Autodesk Inventor part; units mm, degrees
ref_plane "YZ Plane" through (0, 0, 0) normal (1, 0, 0) x (0, 1, 0)
ref_plane "XZ Plane" through (0, 0, 0) normal (0, 1, 0) x (-1, 0, 0)
ref_plane "XY Plane" through (0, 0, 0) normal (0, 0, 1) x (1, 0, 0)
sketch "Sketch1" plane through (0, 0, 0) normal (0, 1, 0) x (-1, 0, 0)
  line L0 (110, -125) -> (-110, -125)
  line L1 (-110, -125) -> (-110, 125)
  line L2 (-110, 125) -> (110, 125)
  line L3 (110, 125) -> (110, -125)
  line L4 (110, -125) -> (-110, 125) construction
  line L5 (-110, -125) -> (110, 125) construction
  line L6 (-60, 75) -> (60, 75) construction
  line L7 (60, 75) -> (60, -75) construction
  line L8 (60, -75) -> (-60, -75) construction
  line L9 (-60, -75) -> (-60, 75) construction
  line L10 (-60, 75) -> (60, -75) construction
  line L11 (60, 75) -> (-60, -75) construction
  point P0 (0, 0)
  dimension "d0" = 220
  dimension "d1" = 250
  dimension "d2" = 120
  dimension "d3" = 150
extrude "Extrusion1" add sketch "Sketch1" along normal blind 40
hole "Hole1" at (-60, 0, -75) at (60, 0, -75) at (60, 0, 75) at (-60, 0, 75) direction (0, 1, 0) diameter 8 end through all
sketch "Sketch2" plane through (-110, 0, 125) normal (0, 0, 1) x (1, 0, 0)
  line L0 (0, 0) -> (220, 0) construction
  line L1 (0, 40) -> (220, 40) construction
  line L2 (220, 0) -> (0, 40) construction
  line L3 (0, 0) -> (220, 40) construction
  circle A0 centre (110, 20) radius 15
  point P0 (110, 0)
  dimension "d13" = 30
extrude "Extrusion2" cut sketch "Sketch2" against normal through all
properties part number "SACMI DPA TILES GRIP FIXED SUPPORT"
Geometry check sheet. Reference: the model listing, model coordinates, mm. Coordinates: 2 decimals unless noted, no trailing zeros. Order: outer loops, then holes, each group sorted by start corner. A loop starts at its lowest first (then second) coordinate and runs counter-clockwise, first axis right, second up. Notation, with made-up numbers: (-31.5, 32.25) -> (18.5, 32.25) arc R26 ccw to (18.5, 49.25) -> close; hole circle Ø2 at (30.25, 18.25). An arc over 180 degrees is marked (long way). Use a Markdown table: item, result. Add a question column.
1. Cross-section at A-A (y = 20). Enter the section's corners in (x, z).
2. Cross-section at B-B (z = 75). Enter the section's corners in (x, y), and give its area (3 significant figures).
3. Mould release check, pull along X, two halves, no side actions. Record for faces 1 (the face through (2, 40, 2)), 2 (the face through (63.905, 20.28, -74.133)), 3 (the face through (-110, 20, 2)): pulls with the +X half, pulls with the -X half, needs draft (parallel to the pull), parting line crosses it, or undercut.
4. Cross-section at C-C (x = -60). Enter the section's corners in (y, z).
5. Cross-section at D-D (x = 0). Enter the section's corners in (y, z).
6. Go/stop test with flat-tipped pins: pin 1 Ø10.5 at (x, z) = (-60, -75) entering from +Y; pin 2 Ø7 at (x, z) = (60, 75) entering from -Y. Record where each tip stops, or that it passes through.
7. Material ranges on L1, parallel to Z at x = -60, y = 23; L2, parallel to X at y = 19, z = 75; L3, parallel to Y at x = 0, z = -73.5, recorded low to high.
Filled sheet:
| question | item | result |
|---|---|---|
| 1 | outline | (-110, -125) -> (-15, -125) -> (-15, 125) -> (-110, 125) -> close; (15, -125) -> (110, -125) -> (110, 125) -> (15, 125) -> close; hole circle Ø8 at (-60, -75); hole circle Ø8 at (-60, 75); hole circle Ø8 at (60, -75); hole circle Ø8 at (60, 75) |
| 2 | outline | (-110, 0) -> (-64, 0) -> (-64, 40) -> (-110, 40) -> close; (-56, 0) -> (56, 0) -> (56, 40) -> (-56, 40) -> close; (64, 0) -> (110, 0) -> (110, 40) -> (64, 40) -> close; hole circle Ø30 at (0, 20) |
| 2 | area | 7,450 mm2 |
| 3 | face 1 | needs draft |
| 3 | face 2 | undercut |
| 3 | face 3 | pulls with the -X half |
| 4 | outline | (0, -125) -> (40, -125) -> (40, -79) -> (0, -79) -> close; (0, -71) -> (40, -71) -> (40, 71) -> (0, 71) -> close; (0, 79) -> (40, 79) -> (40, 125) -> (0, 125) -> close |
| 5 | outline | (0, -125) -> (5, -125) -> (5, 125) -> (0, 125) -> close; (35, -125) -> (40, -125) -> (40, 125) -> (35, 125) -> close |
| 6 | pin 1 | y = 40 |
| 6 | pin 2 | through |
| 7 | L1 | -125 to -79, -71 to 71, 79 to 125 |
| 7 | L2 | -110 to -64, -56 to -14.97, 14.97 to 56, 64 to 110 |
| 7 | L3 | 0 to 5, 35 to 40 |
